Part model, mm, in its own coordinate system. Face numbers are marked on the shaded views. Coordinates: 2 decimals unless noted, no trailing zeros. Loops run counter-clockwise (first coordinate to the right, second up) from the corner with the lowest first, then second, coordinate; pieces in that order, holes last.
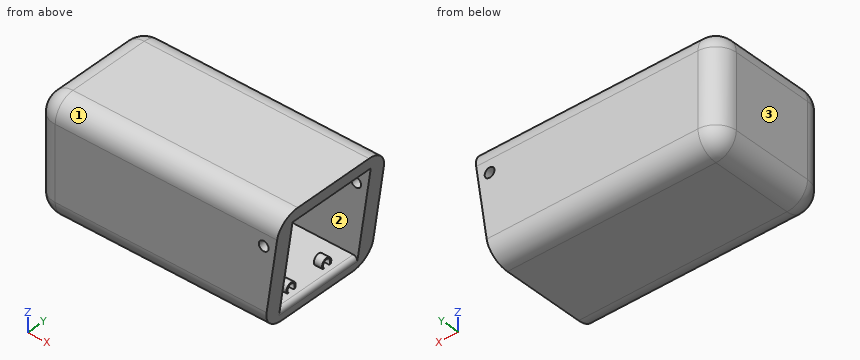
```python
from build123d import *

# Parameters (mm, degrees)
F0_W           = 30
F0_H           = 14
F1_DEPTH       = 15
F2_W           = 11
F2_H           = 11
F3_DEPTH       = 28
F5_R           = 0.65
F5_R_2         = 0.5
F6_DEPTH       = 1
F8_DEPTH       = 25
F9_R           = 2.5
F10_R          = 0.6
F11_DEPTH      = 20
F13_R          = 0.65
F13_R_2        = 0.5
F14_DEPTH      = 1
F15_R          = 0.5
F17_R          = 0.65
F17_R_2        = 0.5
F18_DEPTH      = 0.5
F18_DEPTH_BACK = 0.5
F19_R          = 0.65
F19_R_2        = 0.5
F20_DEPTH      = 1


with BuildPart() as f1:
    # F0 (on Front) → F1 (new body)
    with BuildSketch(Plane.XZ):
        Rectangle(F0_W, F0_H)
    extrude(amount=F1_DEPTH)

    # F2 (on face) → F3 (cut)
    with BuildSketch(Plane.YZ.offset(15)):
        with Locations((-7.5, 0)):
            Rectangle(F2_W, F2_H)
    extrude(amount=-F3_DEPTH, mode=Mode.SUBTRACT)

    # F5 (on offset) → F6 (join)
    with BuildSketch(Plane.YZ.offset(12)):
        with Locations((-10, -5.15)):
            Circle(F5_R)
        with Locations((-10, -5.15)):
            Circle(F5_R_2, mode=Mode.SUBTRACT)
        with Locations((-5, -5.15)):
            Circle(F5_R)
        with Locations((-5, -5.15)):
            Circle(F5_R_2, mode=Mode.SUBTRACT)
    extrude(amount=-F6_DEPTH)

    # F7 (on face) → F8 (cut)
    with BuildSketch(Plane(origin=(0, 0, 0), x_dir=(-1, 0, 0), z_dir=(0, 1, 0))):
        Polygon((-13, -7), (-15, 7), (-15, -7), align=None)
    extrude(amount=-F8_DEPTH, mode=Mode.SUBTRACT)

    # F9
    f9_edges = [f1.edges().sort_by_distance(p)[0] for p in [
        (0, 0, 7),
        (0, -15, 7),
        (-1, 0, -7),
        (-15, -7.5, 7),
        (-15, -7.5, -7),
        (-15, 0, 0),
        (-15, -15, 0),
        (-1, -15, -7),
    ]]
    fillet(f9_edges, radius=F9_R)

    # F10 (on face) → F11 (cut)
    with BuildSketch(Plane.XZ.offset(15)):
        with Locations((13, 3)):
            Circle(F10_R)
    extrude(amount=-F11_DEPTH, mode=Mode.SUBTRACT)

    # F13 (on offset) → F14 (join)
    with BuildSketch(Plane.YZ.offset(-10)):
        with Locations((-10, -5.15)):
            Circle(F13_R)
        with Locations((-10, -5.15)):
            Circle(F13_R_2, mode=Mode.SUBTRACT)
        with Locations((-5, -5.15)):
            Circle(F13_R)
        with Locations((-5, -5.15)):
            Circle(F13_R_2, mode=Mode.SUBTRACT)
    extrude(amount=F14_DEPTH)

    # F15
    f15_edges = [f1.edges().sort_by_distance(p)[0] for p in [
        (13.214286, -7.5, -5.5),
    ]]
    fillet(f15_edges, radius=F15_R)

    # F17 (on offset) → F18 (join, two sides)
    with BuildSketch(Plane.YZ.offset(8)) as f18_sk:
        with Locations((-10, 5.15)):
            Circle(F17_R)
        with Locations((-10, 5.15)):
            Circle(F17_R_2, mode=Mode.SUBTRACT)
        with Locations((-5, 5.15)):
            Circle(F17_R)
        with Locations((-5, 5.15)):
            Circle(F17_R_2, mode=Mode.SUBTRACT)
    extrude(amount=F18_DEPTH)
    extrude(f18_sk.sketch, amount=-F18_DEPTH_BACK)

    # F19 (on offset) → F20 (join)
    with BuildSketch(Plane.YZ.offset(-10)):
        with Locations((-10, 5.15)):
            Circle(F19_R)
        with Locations((-10, 5.15)):
            Circle(F19_R_2, mode=Mode.SUBTRACT)
        with Locations((-5, 5.15)):
            Circle(F19_R)
        with Locations((-5, 5.15)):
            Circle(F19_R_2, mode=Mode.SUBTRACT)
    extrude(amount=F20_DEPTH)


solid = f1.part
```
Q1. Saw through at A-A (x = -2.5). List the corners of the cut face in (y, z), plus the area to 3 significant figures.
Q2. Drop flat-ended pins along their axis: P1, Ø0.8, axis at y = -5, z = 5, coming from the +X side; P2, Ø0.5, axis at y = -5, z = -5, coming from the -X side; P3, Ø0.8, axis at y = -9.5, z = -5, coming from the +X side. Give the stop position or say it passes through.
Q3. Saw through at D-D (z = 1). List the corners of the cut face in (x, y).
Q4. Saw through at C-C (y = -5). List the corners of the cut face in (x, z), plus the area to 3 significant figures.
Q5. Mould opens along Z. For the marked faces 1, 2 and 3 say: released by +Z, released by -Z, zero draft, split by the parting line, or undercut.
Q6. Saw through at B-B (z = 3). List the corners of the cut face in (x, y), plus the area to 3 significant figures.
Q7. Probe line 1 (Z direction, x = -4.5, y = -5.75); line 2 (Y direction, x = 11.35, z = -5.15); line 3 (Y direction, x = 0, z = 4). List the from-to ranges inside material, lowest first.
Checked values:
1. outline: (-15, -4.5) arc R2.5 ccw to (-12.5, -7) - (-2.5, -7) arc R2.5 ccw to (0, -4.5) - (0, 4.5) arc R2.5 ccw to (-2.5, 7) - (-12.5, 7) arc R2.5 ccw to (-15, 4.5) - close; hole (-13, -5.5) - (-2, -5.5) - (-2, 5.5) - (-13, 5.5) - close
1. area: 83.6 mm2
2. P1: stops at x = 8.5
2. P2: stops at x = -14.99
2. P3: stops at x = 12
3. outline: (-15, -12.5) arc R2.5 ccw to (-12.5, -15) - (14.14, -15) - (14.14, -13) - (-13, -13) - (-13, -2) - (14.14, -2) - (14.14, 0) - (-12.5, 0) arc R2.5 ccw to (-15, -2.5) - close
4. outline: (-15, -4.5) arc R2.5 ccw to (-12.5, -7) - (13, -7) - (13.13, -6.07) arc R0.5 ccw to (12.64, -5.5) - (-13, -5.5) - (-13, 5.5) - (14.79, 5.5) - (15, 7) - (-12.5, 7) arc R2.5 ccw to (-15, 4.5) - close; (-10, -4.65) - (-9, -4.65) - (-9, -4.5) - (-10, -4.5) - close; (-10, 4.5) - (-9, 4.5) - (-9, 4.65) - (-10, 4.65) - close; (7.5, 4.5) - (8.5, 4.5) - (8.5, 4.65) - (7.5, 4.65) - close; (11, -4.65) - (12, -4.65) - (12, -4.5) - (11, -4.5) - close
4. area: 107 mm2
5. face 1: released by +Z
5. face 2: undercut
5. face 3: zero draft
6. outline: (-15, -12.5) arc R2.5 ccw to (-12.5, -15) - (12.4, -15) - (12.4, -13) - (-13, -13) - (-13, -2) - (12.4, -2) - (12.4, 0) - (-12.5, 0) arc R2.5 ccw to (-15, -2.5) - close; (13.6, -15) - (14.43, -15) - (14.43, -13) - (13.6, -13) - close; (13.6, -2) - (14.43, -2) - (14.43, 0) - (13.6, 0) - close
6. area: 132 mm2
7. line 1: z = -7 to -5.5, 5.5 to 7
7. line 2: y = -14.91 to -13, -10.65 to -10.5, -9.5 to -9.35, -5.65 to -5.5, -4.5 to -4.35, -2 to -0.09
7. line 3: y = -15 to -13, -2 to 0
